Autodesk Inventor part; units mm, degrees
ref_plane "YZ Plane" through (0, 0, 0) normal (1, 0, 0) x (0, 1, 0)
ref_plane "XZ Plane" through (0, 0, 0) normal (0, 1, 0) x (-1, 0, 0)
ref_plane "XY Plane" through (0, 0, 0) normal (0, 0, 1) x (1, 0, 0)
sketch "スケッチ1" plane through (0, 0, 0) normal (0, 1, 0) x (-1, 0, 0)
  circle A0 centre (0, 0) radius 25
  dimension "d0" = 50
extrude "押し出し1" add sketch "スケッチ1" along normal blind 5
sketch "スケッチ4" plane through (0, 5, 0) normal (0, 1, 0) x (1, 0, 0)
  circle A0 centre (0, 0) radius 17.5
  dimension "d9" = 35
extrude "押し出し4" cut sketch "スケッチ4" against normal through all
sketch "スケッチ8" plane through (0, 5, 0) normal (0, 1, 0) x (1, 0, 0)
  circle A0 centre (0, 0) radius 17.5
  circle A1 centre (0, 17.5) radius 4
  circle A2 centre (-15.1554, -8.75) radius 4
  circle A3 centre (15.1554, -8.75) radius 4
  point P0 (-12.7727, -11.9628)
  point P1 (-16.7464, -5.08)
  point P2 (12.7727, -11.9628)
  point P3 (16.7464, -5.08)
  point P4 (3.9738, 17.0429)
  point P5 (-3.9738, 17.0429)
  dimension "d43" = 8
  dimension "d46" = 360
extrude "押し出し8" cut sketch "スケッチ8" against normal through all contours A0 A1 | A3 A0 | A0 A2 picked at (-0.0763, 18.7972) picked at (16.3019, -9.3615) picked at (-16.2807, -9.3997)
fillet "フィレット2" radius 2 6 edges at (-16.7464, 2.5, 5.08) (-12.7727, 2.5, 11.9628) (3.9738, 2.5, -17.0429) (-3.9738, 2.5, -17.0429) (16.7464, 2.5, 5.08) (12.7727, 2.5, 11.9628)
chamfer "面取り2" distance 0.5 angle 45 26 edges at (25, 5, 0) (15.1554, 5, -8.75) (-15.1554, 5, -8.75) (0, 5, 17.5) (17.1506, 5, 4.8202) (12.7497, 5, 12.4427) (18.6195, 5, 10.75) (-17.1506, 5, 4.8202) (-12.7497, 5, 12.4427) (-18.6195, 5, 10.75) (4.4009, 5, -17.263) (-4.4009, 5, -17.263) (0, 5, -21.5) (-15.1554, 0, -8.75) (-17.1506, 0, 4.8202) (-12.7497, 0, 12.4427) (-18.6195, 0, 10.75) (15.1554, 0, -8.75) (0, 0, 17.5) (17.1506, 0, 4.8202) (12.7497, 0, 12.4427) (18.6195, 0, 10.75) (4.4009, 0, -17.263) (-4.4009, 0, -17.263) (0, 0, -21.5) (25, 0, 0)
properties part number "B_probe_bearing_clamp" material "PAEK 樹脂"
Here's how the part is built. I have some questions about the finished solid (model axes, mm). A direction names the side the tool comes from. Coordinates: 2 decimals unless noted, no trailing zeros. Write each loop counter-clockwise with the first axis right and the second up, starting at its lowest first coordinate (ties: lowest second). Pieces come first, ordered by that corner, then holes.
Item 1: Will these pins go through, and if not, where does the flat tip stop? pin 1 (3 mm diameter, centred on y = 3.5, z = -13, fed in from -X); pin 2 (3 mm diameter, centred on x = -8, z = -15, fed in from +Y); pin 3 (3 mm diameter, centred on x = 19, y = 2.5, fed in from -Z); pin 4 (3 mm diameter, centred on x = 16, y = 2.5, fed in from +Z).
Item 2: If I drill on line 1 (X direction, y = 3.5, z = 0.5) (3 decimals); line 2 (Z direction, x = 8, y = 3.4); line 3 (X direction, y = 1.95, z = 4.5), over which ranges is the centre line in solid material (lowest first)?
Item 3: If we mould it in two halves opening along X, with no side actions, what happens to faces 5 (the cylindrical face through (18.58, 2.53, 10.82)), 6 (the flat face through (4, 0, 18))? For each: +X half, -X half, draft (parallel to the pull), parting line (faces both ways), or undercut.
Item 4: I want a section at B-B on x = 0. Write out the boundary of the cut face in (y, z), and give its area (3 significant figures).
Item 5: On a 3-axis mill with a long thin cutter (end or side, diameter ignored), from which of +Z, -Z, +X, -X, +Y, -Y can I reach the whole of each face in a straight line? I mean faces 1 (the flat face through (4, 5, 18)), 2 (the cylindrical face through (0.1, 2.5, -21.5)), 3 (the conical face through (-15.37, 0.36, -8.66)), 4 (the conical face through (-0.18, 4.64, 17.64)). Say none if no direction works.
Item 6: I want a section at A-A on z = 0. Write out the boundary of the cut face in (x, y).
Findings below:
1. pin 1: stops at x = -22.2
1. pin 2: stops at y = 5
1. pin 3: stops at z = -17.85
1. pin 4: stops at z = 20.37
2. line 1: x = -24.995 to -17.493, 17.493 to 24.995
2. line 2: z = -23.69 to -15.56, 15.56 to 23.69
2. line 3: x = -24.59 to -17.07, 17.07 to 24.59
3. face 5: undercut
3. face 6: draft
4. outline: (0, -24.5) - (0.5, -25) - (4.5, -25) - (5, -24.5) - (5, -22) - (4.5, -21.5) - (0.5, -21.5) - (0, -22) - close; (0, 18) - (0.5, 17.5) - (4.5, 17.5) - (5, 18) - (5, 24.5) - (4.5, 25) - (0.5, 25) - (0, 24.5) - close
4. area: 54.0 mm2
5. face 1: +Z, -Z, +X, -X, +Y
5. face 2: +Y, -Y
5. face 3: -Y
5. face 4: +Y
6. outline: (-25, 0.5) - (-24.5, 0) - (-18, 0) - (-17.5, 0.5) - (-17.5, 4.5) - (-18, 5) - (-24.5, 5) - (-25, 4.5) - close; (17.5, 0.5) - (18, 0) - (24.5, 0) - (25, 0.5) - (25, 4.5) - (24.5, 5) - (18, 5) - (17.5, 4.5) - close
